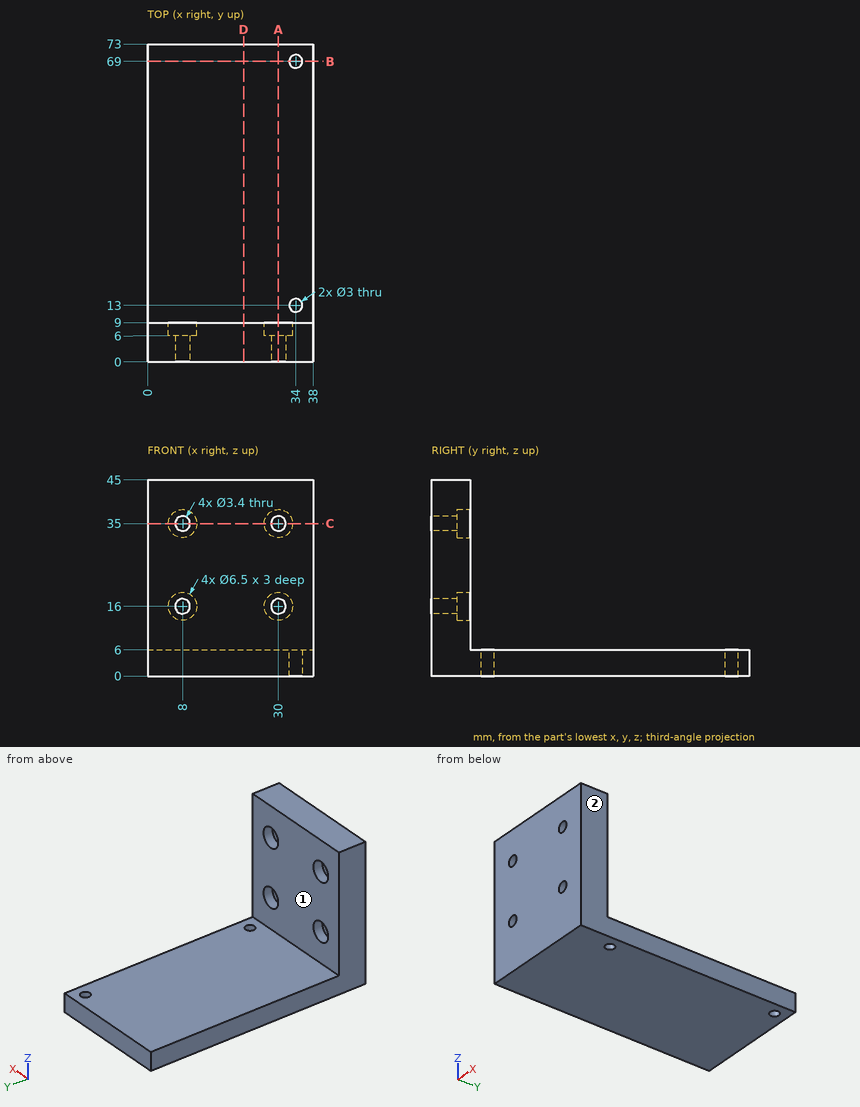
Can you work these out from the drawing? Everything is in mm from the part's minimum corner. A direction names the side the tool comes from. Coordinates: 2 decimals unless noted, no trailing zeros. Write each loop counter-clockwise with the first axis right and the second up, starting at its lowest first coordinate (ties: lowest second). Pieces come first, ordered by that corner, then holes. Notation, with made-up numbers: (65, 63) -> (72, 63) arc R22 cw to (72, 72) -> close; hole circle Ø5 at (50.5, 49). An arc over 180 degrees is marked (long way). Return JSON: item names as keys, results as strings.
(1) Imagine slicing it at B-B, the plane y = 69. Please give me the cut outline in (x, z).
Numbers:
{"outline": "(0, 0) -> (32.5, 0) -> (32.5, 6) -> (0, 6) -> close; (35.5, 0) -> (38, 0) -> (38, 6) -> (35.5, 6) -> close"}
(2) Imagine slicing it at D-D, the plane x = 22. Please give me the cut outline in (y, z), then the cut area to 3 significant figures.
Numbers:
{"outline": "(0, 0) -> (73, 0) -> (73, 6) -> (9, 6) -> (9, 45) -> (0, 45) -> close", "area": "789 mm2"}
(3) Which directions (+Z, -Z, +X, -X, +Y, -Y) give clear straight access to the entire face, cutting with the end or side of a thin tool? Please do the marked faces 1 and 2.
Numbers:
{"face 1": "+Z, +X, -X, +Y", "face 2": "+Z, -Z, +X, +Y, -Y"}
(4) I need wall thicknesses on L1, parallel to X at y = 6.95, z = 16; L2, parallel to Y at x = 34, z = 4.55; L3, parallel to X at y = 4, z = 35. Which ranges of each line are inside material? Lowest first, please.
Numbers:
{"L1": "x = 0 to 4.75, 11.25 to 26.75, 33.25 to 38", "L2": "y = 0 to 11.5, 14.5 to 67.5, 70.5 to 73", "L3": "x = 0 to 6.3, 9.7 to 28.3, 31.7 to 38"}
(5) Imagine slicing it at C-C, the plane z = 35. Please give me the cut outline in (x, y), then the cut area to 3 significant figures.
Numbers:
{"outline": "(0, 0) -> (6.3, 0) -> (6.3, 6) -> (4.75, 6) -> (4.75, 9) -> (0, 9) -> close; (9.7, 0) -> (28.3, 0) -> (28.3, 6) -> (26.75, 6) -> (26.75, 9) -> (11.25, 9) -> (11.25, 6) -> (9.7, 6) -> close; (31.7, 0) -> (38, 0) -> (38, 9) -> (33.25, 9) -> (33.25, 6) -> (31.7, 6) -> close", "area": "262 mm2"}
(6) Imagine slicing it at A-A, the plane x = 30. Please give me the cut outline in (y, z).
Numbers:
{"outline": "(0, 0) -> (73, 0) -> (73, 6) -> (9, 6) -> (9, 12.75) -> (6, 12.75) -> (6, 14.3) -> (0, 14.3) -> close; (0, 17.7) -> (6, 17.7) -> (6, 19.25) -> (9, 19.25) -> (9, 31.75) -> (6, 31.75) -> (6, 33.3) -> (0, 33.3) -> close; (0, 36.7) -> (6, 36.7) -> (6, 38.25) -> (9, 38.25) -> (9, 45) -> (0, 45) -> close"}
(7) I'm going to push flat-ended pins straight in: pin 1 (8 mm diameter, centred on x = 23.5, z = 14.5, fed in from +Y); pin 2 (4 mm diameter, centred on x = 30, z = 16, fed in from +Y); pin 3 (8 mm diameter, centred on x = 13, y = 14.5, fed in from +Z); pin 4 (8.5 mm diameter, centred on x = 8, z = 35, fed in from -Y). Where does each tip first touch, or does it pass through?
Numbers:
{"pin 1": "stops at y = 9", "pin 2": "stops at y = 6", "pin 3": "stops at z = 6", "pin 4": "stops at y = 0"}
